Autodesk Inventor part; units mm, degrees
ref_plane "YZ Plane" through (0, 0, 0) normal (1, 0, 0) x (0, 1, 0)
ref_plane "XZ Plane" through (0, 0, 0) normal (0, 1, 0) x (-1, 0, 0)
ref_plane "XY Plane" through (0, 0, 0) normal (0, 0, 1) x (1, 0, 0)
sketch "Sketch1" plane through (0, 0, 0) normal (0, 0, 1) x (1, 0, 0)
  arc A0 (-1.325, -1.5313) -> (-1.325, 1.5313) centre (0, 0) ccw
  line L0 (-1.325, -1.5313) -> (-1.325, 1.5313)
  arc A1 (4, 0) -> (2.6774, -2.9718) centre (0, 0) ccw
  line L1 (2.6774, -2.9718) -> (88.9, -2.9718)
  line L2 (88.9, -2.9718) -> (88.9, 0)
  line L3 (88.9, 0) -> (4, 0)
  dimension "d0" = 4.05
  dimension "d2" = 8
  dimension "d3" = 3.35
  dimension "d5" = 88.9
  dimension "d7" = 2.9718
  dimension "d8" = 84.9
extrude "Extrusion1" add sketch "Sketch1" along normal blind 9.398
properties part number "Rotator2"
CAD build for the part. Positions are in the model's coordinates, mm. A direction names the side the tool comes from. Round coordinates to 2 decimals unless told otherwise and drop trailing zeros. Write each loop counter-clockwise with the first axis right and the second up, starting at its lowest first coordinate (ties: lowest second). Pieces come first, ordered by that corner, then holes.
Item 1: Tool access for faces 1 (the flat face through (47, 0, 5)), 2 (the flat face through (45, -2.972, 5)), 3 (the cylindrical face through (-3.71, 1.49, 4.63)): list every direction of +Z, -Z, +X, -X, +Y, -Y with a clear straight run to the whole face (end or side of a thin tool).
Filled in:
face 1: +Z, -Z, +X, +Y
face 2: +Z, -Z, +X, -Y
face 3: +Z, -Z
Item 2: Band-saw the part on A-A on x = 0. Write the cut outline in (y, z).
Filled in:
outline: (-4, 0) - (-2.02, 0) - (-2.02, 9.4) - (-4, 9.4) - close; (2.02, 0) - (4, 0) - (4, 9.4) - (2.02, 9.4) - close
Item 3: Drop flat-ended pins along their axis: pin 1 Ø1 at (y, z) = (2, 6) entering from -X; pin 2 Ø1.5 at (y, z) = (1, 1.5) entering from +X; pin 3 Ø5 at (x, z) = (69.5, 1) entering from +Y. Give the stop position or say it passes through.
Filled in:
pin 1: stops at x = -3.71
pin 2: stops at x = 3.99
pin 3: stops at y = 0
Item 4: Mould opens along X. For faces 4 (the flat face through (88.9, -2, 5)), 5 (the flat face through (39, -2, 9.398)), 6 (the flat face through (-1.325, 0, 5)) say: released by +X, released by -X, zero draft, split by the parting line, or undercut.
Filled in:
face 4: released by +X
face 5: zero draft
face 6: undercut
Item 5: Band-saw the part on B-B on z = 7.25. Write the cut outline in (x, y) (3 decimals).
Filled in:
outline: (2.677, -2.972) - (88.9, -2.972) - (88.9, 0) - (4, 0) arc R4 ccw (long way) to start; hole (-1.325, -1.531) arc R2.025 ccw (long way) to (-1.325, 1.531) - close
Item 6: Band-saw the part on C-C on x = 66. Write the cut outline in (y, z), then the cut area to 3 significant figures.
Filled in:
outline: (-2.97, 0) - (0, 0) - (0, 9.4) - (-2.97, 9.4) - close
area: 27.9 mm2
Item 7: Drill centre lines: L1, parallel to Y at x = 0, z = 5.25; L2, parallel to Y at x = 36, z = 1.25; L3, parallel to X at y = 0.5, z = 9 (3 decimals). Where is each one in solid material? Low to high.
Filled in:
L1: y = -4 to -2.02, 2.02 to 4
L2: y = -2.97 to 0
L3: x = -3.969 to -1.325, 1.962 to 3.969
